```python
from build123d import *

# Parameters (mm, degrees)
SZKIC1_R                    = 11
SZKIC1_W                    = 15.5
SZKIC1_H                    = 5
DODANIE_WYCI_GNI_CIE1_DEPTH = 2


with BuildPart() as part:
    # Szkic1 → Dodanie-wyciągnięcie1 (new body)
    with BuildSketch(Plane(origin=(0, 0, 0), x_dir=(1, 0, 0), z_dir=(0, 1, 0))):
        with Locations(Location((0, 0, 0), (0, 0, 270))):
            Circle(SZKIC1_R)
        Rectangle(SZKIC1_W, SZKIC1_H, mode=Mode.SUBTRACT)
    extrude(amount=DODANIE_WYCI_GNI_CIE1_DEPTH)


solid = part.part
```
For this review, take the finished solid that the model builds, in its own axes (mm). A direction names the side the tool comes from. Coordinates: 2 decimals unless noted, no trailing zeros. Write each loop counter-clockwise with the first axis right and the second up, starting at its lowest first coordinate (ties: lowest second). Pieces come first, ordered by that corner, then holes. Notation, with made-up numbers: (37, 68) - (53, 68) arc R28 cw to (53, 96) - close; hole circle Ø9 at (56.25, 9). An arc over 180 degrees is marked (long way). Answer in a Markdown table with one row per item. Add a question column.
Q1. Tool access review of faces 1 (the flat face through (0, 0, -3)), 2 (the flat face through (7.75, 1, 0)): name each direction out of +Z, -Z, +X, -X, +Y, -Y from which nothing blocks a thin tool from reaching the whole face with its end or side.
Q2. We need section D-D, the plane z = 7.75. State the section outline as (x, y) points.
Q3. We need section A-A, the plane x = -7. State the section outline as (y, z) points, and give its area (3 significant figures).
Q4. For probe 1 along X at (y, z) = (1, 0); probe 2 along Z at (x, y) = (-5.75, 1.1); probe 3 along Z at (x, y) = (3, 1.1), list the stretches that pass through material, from the lowest coordinate up.
Q5. Draft analysis for pull direction Z (two halves, no side actions). For faces 3 (the flat face through (0, 2, -3)), 4 (the flat face through (-7.75, 1, 0)), 5 (the cylindrical face through (-10.74, 0.99, -2.38)), state which applies: +Z half, -Z half, draft (parallel to the pull), parting line (faces both ways), or undercut.
Q6. For P1, Ø5, axis at x = -6, z = 5, coming from the -Y side; P2, Ø0.6, axis at x = -1.5, y = 1, coming from the -Z side; P3, Ø1, axis at x = -6.5, y = 0.5, coming from the +Z side; P4, Ø0.6, axis at x = -1.5, y = 0.5, coming from the +Z side, all flat-tipped, find the tip position at first contact; note any pin that passes through.
Q7. We need section C-C, the plane y = 1. State the section outline as (x, z) points, and give its area (3 significant figures).
Q8. We need section B-B, the plane z = 0. State the section outline as (x, y) points, and give its area (3 significant figures).
Answer list:
| question | item | result |
|---|---|---|
| 1 | face 1 | +Z, -Z, +X, -X, -Y |
| 1 | face 2 | +Y, -Y |
| 2 | outline | (-7.81, 0) - (7.81, 0) - (7.81, 2) - (-7.81, 2) - close |
| 3 | outline | (0, -8.49) - (2, -8.49) - (2, -2.5) - (0, -2.5) - close; (0, 2.5) - (2, 2.5) - (2, 8.49) - (0, 8.49) - close |
| 3 | area | 23.9 mm2 |
| 4 | probe 1 | x = -11 to -7.75, 7.75 to 11 |
| 4 | probe 2 | z = -9.38 to -2.5, 2.5 to 9.38 |
| 4 | probe 3 | z = -10.58 to -2.5, 2.5 to 10.58 |
| 5 | face 3 | draft |
| 5 | face 4 | undercut |
| 5 | face 5 | parting line |
| 6 | P1 | stops at y = 0 |
| 6 | P2 | stops at z = -10.93 |
| 6 | P3 | stops at z = 9.22 |
| 6 | P4 | stops at z = 10.93 |
| 7 | outline | circle Ø22 at (0, 0); hole (-7.75, -2.5) - (7.75, -2.5) - (7.75, 2.5) - (-7.75, 2.5) - close |
| 7 | area | 303 mm2 |
| 8 | outline | (-11, 0) - (-7.75, 0) - (-7.75, 2) - (-11, 2) - close; (7.75, 0) - (11, 0) - (11, 2) - (7.75, 2) - close |
| 8 | area | 13.0 mm2 |
